```python
from build123d import *

# Parameters (mm, degrees)
F0_W     = 10
F0_H     = 40
F1_DEPTH = 140
F2_R     = 7
F3_DEPTH = 10.001
F4_W     = 80
F4_H     = 40
F4_R     = 6
F4_W_2   = 40
F5_DEPTH = 10
F7_DEPTH = 10


# Not quite as in the source:
# - a feature names something its author has since deleted; it is built from what else it names


with BuildPart() as f1:
    # F0 (on Right) → F1 (new body)
    with BuildSketch(Plane.YZ):
        Rectangle(F0_W, F0_H)
    extrude(amount=-F1_DEPTH)

    # F2 (on face) → F3 (cut, through all)
    with BuildSketch(Plane.XZ.offset(5)):
        with Locations((-120, 0)):
            Circle(F2_R)
    extrude(amount=-F3_DEPTH, mode=Mode.SUBTRACT)

    # F4 (on face) → F5 (join)
    with BuildSketch(Plane.XZ.offset(5)):
        with Locations((40, 0)):
            Rectangle(F4_W, F4_H)
        with Locations((60, 0)):
            Circle(F4_R, mode=Mode.SUBTRACT)
        with Locations((-20, 0)):
            Rectangle(F4_W_2, F4_H)
    extrude(amount=F5_DEPTH)

    # F6 (on face) → F7 (cut, through all)
    with BuildSketch(Plane(origin=(0, 5, 0), x_dir=(-1, 0, 0), z_dir=(0, 1, 0))):
        Polygon((15, -20), (0, -5), (0, -20), align=None)
    extrude(amount=-F7_DEPTH, mode=Mode.SUBTRACT)


solid = f1.part
```
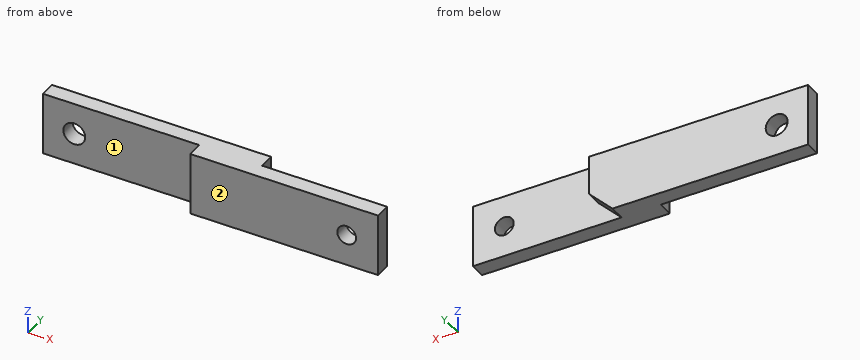
Geometry check sheet. Reference: the model listing, model coordinates, mm. Face numbers are marked on the shaded views. A direction names the side the tool comes from. Coordinates: 2 decimals unless noted, no trailing zeros. Write each loop counter-clockwise with the first axis right and the second up, starting at its lowest first coordinate (ties: lowest second). Pieces come first, ordered by that corner, then holes. Notation, with made-up numbers: (76.25, 32) -> (113.25, 32) arc R20 ccw to (113.25, 55) -> close; hole circle Ø10 at (-17.5, 47.5). An arc over 180 degrees is marked (long way). Use CSV: the item, a comma, the result in double quotes. Start each with the question number.
Item 1: Cross-section at C-C, the plane y = 0. Record the cut outline in (x, z).
Item 2: Cross-section at D-D, the plane z = -12.5. Record the cut outline in (x, y), plus the area to 4 significant figures.
Item 3: Cross-section at A-A, the plane z = 0. Record the cut outline in (x, y).
Item 4: Depth check by flat-ended pin: pin 1 Ø2 at (x, z) = (-110, -1.5) entering from -Y; pin 2 Ø8 at (y, z) = (1, -3.5) entering from +X; pin 3 Ø1.5 at (y, z) = (-10, -13.5) entering from -X; pin 4 Ø7 at (x, z) = (60, 0) entering from -Y. Enter the tip coordinate at first touch or a pass-through.
Item 5: Set-up check for the marked faces 1 and 2: record each of +Z, -Z, +X, -X, +Y, -Y from which the full face is reachable in a straight line by a thin tool's end or side.
Item 6: Cross-section at B-B, the plane x = -120. Record the cut outline in (y, z), plus the area to 3 significant figures.
Item 7: Thickness scan on line 1 (Z direction, x = 60, y = -8); line 2 (Z direction, x = -120, y = 0.75); line 3 (X direction, y = -8.25, z = -17). Record the ranges inside material, lowest first.
Answers:
1,outline,"(-140, -20) -> (-15, -20) -> (0, -5) -> (0, 20) -> (-140, 20) -> close; hole circle Ø14 at (-120, 0)"
2,outline,"(-140, -5) -> (-40, -5) -> (-40, -15) -> (80, -15) -> (80, -5) -> (-7.5, -5) -> (-7.5, 5) -> (-140, 5) -> close"
2,area,"2,525 mm^2"
3,outline,"(-140, -5) -> (-127, -5) -> (-127, 5) -> (-140, 5) -> close; (-113, -5) -> (-40, -5) -> (-40, -15) -> (54, -15) -> (54, -5) -> (0, -5) -> (0, 5) -> (-113, 5) -> close; (66, -15) -> (80, -15) -> (80, -5) -> (66, -5) -> close"
4,pin 1,"y = -5"
4,pin 2,"x = 0"
4,pin 3,"x = -40"
4,pin 4,"through"
5,face 1,"+Z, -Z, -X, -Y"
5,face 2,"+Z, -Z, +X, -X, -Y"
6,outline,"(-5, -20) -> (5, -20) -> (5, -7) -> (-5, -7) -> close; (-5, 7) -> (5, 7) -> (5, 20) -> (-5, 20) -> close"
6,area,"260 mm^2"
7,line 1,"-20 to -6, 6 to 20"
7,line 2,"-20 to -7, 7 to 20"
7,line 3,"-40 to 80"
